Answer from the drawing. Dimensions are ordinates in mm from the lowest x, y and z of the part. Round coordinates to 2 decimals unless told otherwise and drop trailing zeros. Loops run counter-clockwise (first coordinate to the right, second up) from the corner with the lowest first, then second, coordinate; pieces in that order, holes last. Notation, with made-up numbers: (-15, 79.25) -> (30, 79.25) arc R27 ccw to (30, 106.25) -> close; hole circle Ø8 at (-9, 62.5). An arc over 180 degrees is marked (long way). One line per question, with ' | ' between items.
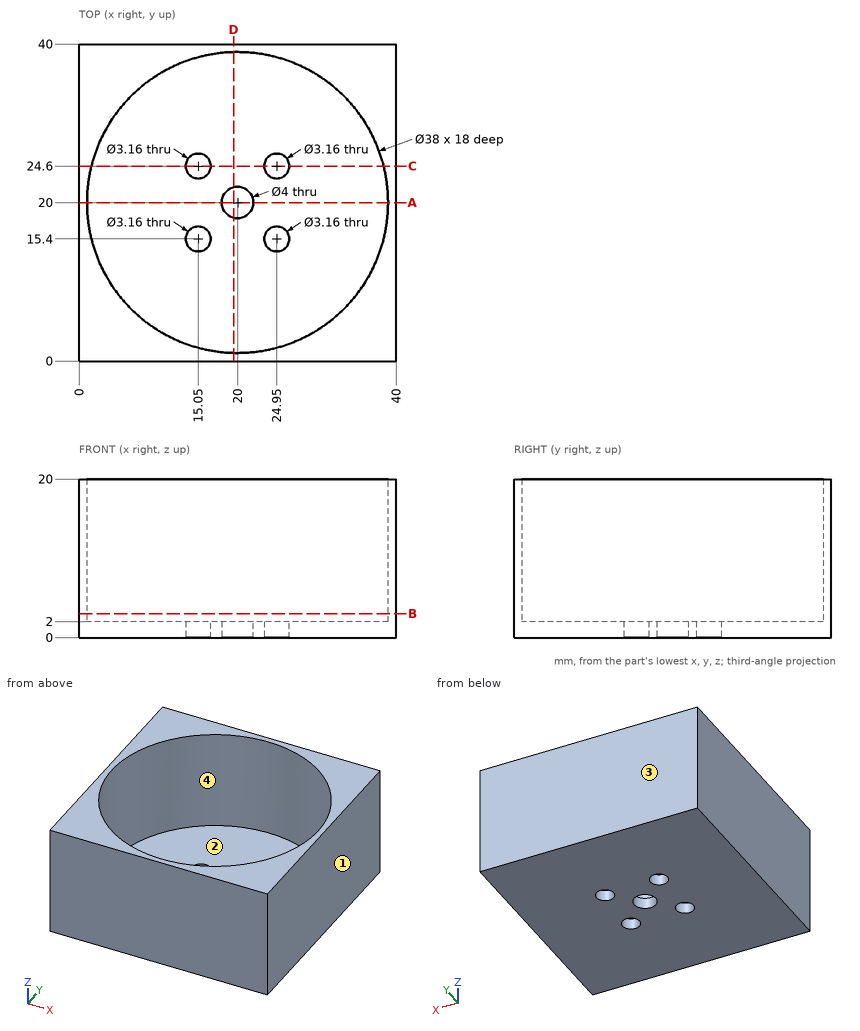
Q1. A cutting plane is placed at C-C on y = 24.6. Give the vertices of the cut face in (x, z), plus the area to 3 significant figures.
Numbers:
outline: (0, 0) -> (13.47, 0) -> (13.47, 2) -> (1.57, 2) -> (1.57, 20) -> (0, 20) -> close; (16.63, 0) -> (23.37, 0) -> (23.37, 2) -> (16.63, 2) -> close; (26.53, 0) -> (40, 0) -> (40, 20) -> (38.43, 20) -> (38.43, 2) -> (26.53, 2) -> close | area: 124 mm^2
Q2. For a pull along Y with two mould halves and no side action, classify the marked faces 1, 2, 3 and 4 as pulls with the +Y half, pulls with the -Y half, needs draft (parallel to the pull), parting line crosses it, or undercut.
Numbers:
face 1: needs draft | face 2: undercut | face 3: pulls with the +Y half | face 4: undercut
Q3. A cutting plane is placed at A-A on y = 20. Give the vertices of the cut face in (x, z).
Numbers:
outline: (0, 0) -> (18, 0) -> (18, 2) -> (1, 2) -> (1, 20) -> (0, 20) -> close; (22, 0) -> (40, 0) -> (40, 20) -> (39, 20) -> (39, 2) -> (22, 2) -> close
Q4. Given pin 1 Ø6.5 at (x, y) = (20, 20) entering from +Z, flat-ended and moving along its own axis, determine where the tip first touches the part or whether it passes through.
Numbers:
pin 1: z = 2
Q5. Find the intervals of material crossed by line 1 (X direction, y = 15.4, z = 0.65); line 2 (Y direction, x = 15.05, z = 0.7); line 3 (Y direction, x = 20, z = 15.25), in increasing order. Write a range as from..to.
Numbers:
line 1: 0..13.47, 16.63..23.37, 26.53..40 | line 2: 0..13.82, 16.98..23.02, 26.18..40 | line 3: 0..1, 39..40
Q6. A cutting plane is placed at B-B on z = 3. Give the vertices of the cut face in (x, y), plus the area to 3 significant figures.
Numbers:
outline: (0, 0) -> (40, 0) -> (40, 40) -> (0, 40) -> close; hole circle Ø38 at (20, 20) | area: 466 mm^2
Q7. A cutting plane is placed at D-D on x = 19.5. Give the vertices of the cut face in (y, z).
Numbers:
outline: (0, 0) -> (18.06, 0) -> (18.06, 2) -> (1.01, 2) -> (1.01, 20) -> (0, 20) -> close; (21.94, 0) -> (40, 0) -> (40, 20) -> (38.99, 20) -> (38.99, 2) -> (21.94, 2) -> close
